The listing builds one solid part. Answer for the finished solid, in the listing's coordinates (mm). A direction names the side the tool comes from. Round coordinates to 2 decimals unless told otherwise and drop trailing zeros. Order: outer loops, then holes, each group sorted by start corner. A loop starts at its lowest first (then second) coordinate and runs counter-clockwise, first axis right, second up. Notation, with made-up numbers: (66.5, 71.5) - (74.5, 71.5) arc R8 cw to (74.5, 79.5) - close; hole circle Ø10 at (76, -7.5). An arc over 180 degrees is marked (long way). Write item = value, one per line.
Autodesk Inventor part; units mm, degrees
ref_plane "YZ Plane" through (0, 0, 0) normal (1, 0, 0) x (0, 1, 0)
ref_plane "XZ Plane" through (0, 0, 0) normal (0, 1, 0) x (-1, 0, 0)
ref_plane "XY Plane" through (0, 0, 0) normal (0, 0, 1) x (1, 0, 0)
sketch "Sketch1" plane through (0, 0, 0) normal (0, 0, 1) x (1, 0, 0)
  line L0 (0, 0) -> (35, 0)
  line L1 (35, 0) -> (35, 35)
  line L2 (35, 35) -> (0, 35)
  line L3 (0, 35) -> (0, 0)
  dimension "d0" = 35
  dimension "d1" = 35
extrude "Extrusion1" add sketch "Sketch1" against normal blind 5
sketch "Sketch2" plane through (0, 0, 0) normal (0, 0, 1) x (1, 0, 0)
  circle A0 centre (12.63, 17.6884) radius 2.425
  circle A1 centre (12.63, 17.6884) radius 1
  point P0 (0, 0)
extrude "Extrusion2" add sketch "Sketch2" along normal blind 3
fillet "Fillet1" radius 0.5 2 edges at (10.205, 17.6884, 3) (11.63, 17.6884, 3)
properties part number "ServoHolderBase"
Q1. Determine the mould class of faces 3 (the face through (11, 17, 3)), 4 (the face through (18, 35, -2)), 5 (the face through (12.413, 18.665, 1.232)) for opening direction Y: released by +Y, released by -Y, zero draft, split by the parting line, or undercut.
Model answer:
face_3 = zero draft
face_4 = released by +Y
face_5 = undercut
Q2. Section C-C on z = 1.5 is taken. Determine the outline of the cut face in (x, y) (3 decimals), then the cut area to 3 significant figures.
Model answer:
outline = circle Ø4.85 at (12.63, 17.688); hole circle Ø2 at (12.63, 17.688)
area = 15.3 mm^2
Q3. Find the intervals of material crossed by line 1 (Y direction, x = 12.63, z = 0.7); line 2 (Z direction, x = 9, y = 26); line 3 (X direction, y = 18.5, z = 2.25), in increasing order. Write a range as from..to.
Model answer:
line_1 = 15.26..16.69, 18.69..20.11
line_2 = -5..0
line_3 = 10.34..12.05, 13.21..14.92
Q4. Section A-A on x = 12.63 is taken. Determine the outline of the cut face in (y, z).
Model answer:
outline = (0, -5) - (35, -5) - (35, 0) - (20.11, 0) - (20.11, 2.5) arc R0.5 ccw to (19.61, 3) - (19.19, 3) arc R0.5 ccw to (18.69, 2.5) - (18.69, 0) - (16.69, 0) - (16.69, 2.5) arc R0.5 ccw to (16.19, 3) - (15.76, 3) arc R0.5 ccw to (15.26, 2.5) - (15.26, 0) - (0, 0) - close
Q5. Section B-B on y = 22 is taken. Determine the outline of the cut face in (x, z), then the cut area to 3 significant figures.
Model answer:
outline = (0, -5) - (35, -5) - (35, 0) - (0, 0) - close
area = 175 mm^2
Q6. For faces 1 (the face through (0, 18, -2)), 2 (the face through (12.314, 15.284, 1.232)), determine the directions among +Z, -Z, +X, -X, +Y, -Y from which every point of the face is accessible in a straight line to the end or side of a thin tool.
Model answer:
face_1 = +Z, -Z, -X, +Y, -Y
face_2 = +Z
Q7. Flat-ended cylindrical pins translate along their axes: P1, Ø10.5, axis at x = 23.5, y = 26, coming from the +Z side; P2, Ø1.6, axis at x = 13, y = 17.5, coming from the +Z side. Find the tip coordinate at first contact, or state that the pin passes through.
Model answer:
P1 = 0
P2 = 2.91
